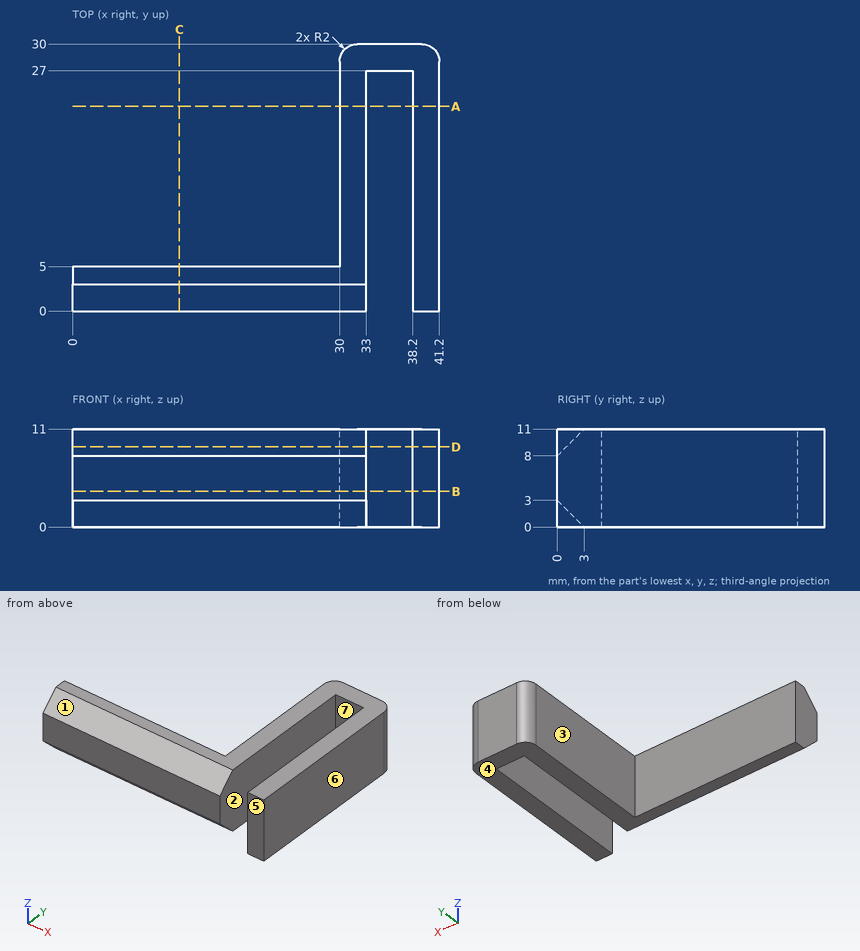
Part print with two shaded views. Sizes in mm from the minimum x, y, z corner. A direction names the side the tool comes from. Give positions to 0.01 mm unless a question says otherwise; leave off trailing zeros. Order: outer loops, then holes, each group sorted by start corner. A loop starts at its lowest first (then second) coordinate and runs counter-clockwise, first axis right, second up.
1) Wall check: probe 1 along X at (y, z) = (17.5, 4); probe 2 along X at (y, z) = (2, 2.25); probe 3 along Y at (x, z) = (17.5, 4). Give the ranges that are in metal, low to high.
2) 3-axis set-ups, long thin cutter, end or side, ignore diameter. For the marked faces 1, 2, 3 and 4: which of +Z, -Z, +X, -X, +Y, -Y reach the whole face in a straight line?
3) Mould opens along X. For the marked faces 5, 6 and 7 say: +X half, -X half, draft (parallel to the pull), parting line (faces both ways), or undercut.
4) Saw through at D-D, the plane z = 9. Write the cut outline in (x, y).
5) Pin check, flat tips, straight feed: pin 1 (3 mm diameter, centred on y = 19, z = 6, fed in from -X); pin 2 (3 mm diameter, centred on x = 14, z = 3, fed in from +Y). Stop position of each tip, or through.
6) Saw through at C-C, the plane x = 12. Write the cut outline in (y, z), then the cut area to 3 significant figures.
7) Saw through at A-A, the plane y = 23. Write the cut outline in (x, z), then the cut area to 3 significant figures.
8) Saw through at B-B, the plane z = 4. Write the cut outline in (x, y).
Computed:
1. probe 1: x = 30 to 33, 38.2 to 41.2
1. probe 2: x = 0 to 33, 38.2 to 41.2
1. probe 3: y = 0 to 5
2. face 1: +Z, -X, -Y
2. face 2: +Z, -Z, -Y
2. face 3: +Z, -Z, -X, +Y
2. face 4: -Z, +X, -X, +Y, -Y
3. face 5: draft
3. face 6: +X half
3. face 7: undercut
4. outline: (0, 1) - (33, 1) - (33, 27) - (38.2, 27) - (38.2, 0) - (41.2, 0) - (41.2, 28) arc R2 ccw to (39.2, 30) - (32, 30) arc R2 ccw to (30, 28) - (30, 5) - (0, 5) - close
5. pin 1: stops at x = 30
5. pin 2: stops at y = 5
6. outline: (0, 3) - (3, 0) - (5, 0) - (5, 11) - (3, 11) - (0, 8) - close
6. area: 46.0 mm2
7. outline: (30, 0) - (33, 0) - (33, 11) - (30, 11) - close; (38.2, 0) - (41.2, 0) - (41.2, 11) - (38.2, 11) - close
7. area: 66.0 mm2
8. outline: (0, 0) - (33, 0) - (33, 27) - (38.2, 27) - (38.2, 0) - (41.2, 0) - (41.2, 28) arc R2 ccw to (39.2, 30) - (32, 30) arc R2 ccw to (30, 28) - (30, 5) - (0, 5) - close
